Geometry: final body of the model. Coordinates: model frame, mm. A direction names the side the tool comes from. Coordinates: 2 decimals unless noted, no trailing zeros. Order: outer loops, then holes, each group sorted by start corner. A loop starts at its lowest first (then second) coordinate and runs counter-clockwise, first axis right, second up. Notation, with made-up numbers: M -34.75,5 L 20.25,5 A22 cw 20.25,18 Z; hole C 25,-34.75 d7. An arc over 180 degrees is marked long. Use CSV: the item, a comma, the result in double quotes. Start each with the question number.
Q1. Section query A-A, the plane x = -10. Output: boundary loops of the cut face in (y, z), and give its area (3 significant figures).
Q2. Section query D-D, the plane x = 0. State how many separate pieces and enclosed holes the cut face has, and give its area (3 significant figures).
Q3. Section query C-C, the plane z = -4. Output: boundary loops of the cut face in (x, y), and give its area (3 significant figures).
Q4. First-contact query: P1, Ø0.9, axis at x = 13, z = 0, coming from the +Y side (1 decimal); P2, Ø0.9, axis at x = 1, y = 1.5, coming from the -Z side; P3, Ø2, axis at x = 9, y = 2, coming from the -Z side; P4, Ø13, axis at x = 2.5, z = 13, coming from the -Y side. Flat tips, straight axial feed; report the tip coordinate or a pass-through.
Q5. Ray query, probe 1 along Z at (x, y) = (10, 0.3); probe 2 along Z at (x, y) = (3, 0.55); probe 3 along Y at (x, z) = (16, 3). Return the intervals inside material, ascending.
Q6. Access query for faces 1 (the face through (6, 2, -10)), 2 (the face through (-16.595, 1.371, 0.456)), 3 (the face through (0, 0.75, 14)), 4 (the face through (-1.08, -1.56, 4.88)), 5 (the face through (0, 0.75, -13)). Directions: +Z, -Z, +X, -X, +Y, -Y. A direction counts if a zero-diameter tool reaches every point of the face in a straight line with its end or side. Return the directions, or none.
Q7. Mould query, pull axis Z, two halves, no side actions, for faces 6 (the face through (-13.75, 1.37, -0.03)), 7 (the face through (2.2, -3, -2.2)), 8 (the face through (-0.098, 1.815, -15.744)), 9 (the face through (-22, 1, 0)). Classes: +Z half, -Z half, draft (parallel to the pull), parting line (faces both ways), or undercut.
Q8. Section query B-B, the plane z = 18. Output: boundary loops of the cut face in (x, y), and give its area (3 significant figures).
Autodesk Inventor part; units mm, degrees
ref_plane "YZ Plane" through (0, 0, 0) normal (1, 0, 0) x (0, 1, 0)
ref_plane "XZ Plane" through (0, 0, 0) normal (0, 1, 0) x (-1, 0, 0)
ref_plane "XY Plane" through (0, 0, 0) normal (0, 0, 1) x (1, 0, 0)
sketch "Sketch1" plane through (0, 0, 0) normal (0, 1, 0) x (-1, 0, 0)
  line L0 (6, -15) -> (6, -6)
  line L1 (16, -6) -> (16, 0)
  line L2 (6, -15) -> (0, -15)
  line L3 (16, -6) -> (6, -6)
  arc A0 (0, -21) -> (6, -15) centre (0, -15) ccw
  arc A1 (16, -6) -> (22, 0) centre (16, 0) ccw
  line L4 (6, 15) -> (6, 6)
  line L5 (16, 6) -> (16, 0)
  line L6 (6, 15) -> (0, 15)
  line L7 (16, 6) -> (6, 6)
  arc A2 (6, 15) -> (0, 21) centre (0, 15) ccw
  arc A3 (22, 0) -> (16, 6) centre (16, 0) ccw
  line L8 (-6, -15) -> (-6, -6)
  line L9 (-16, -6) -> (-16, 0)
  line L10 (-6, -15) -> (0, -15)
  line L11 (-16, -6) -> (-6, -6)
  arc A4 (-6, -15) -> (0, -21) centre (0, -15) ccw
  arc A5 (-22, 0) -> (-16, -6) centre (-16, 0) ccw
  line L12 (-16, 6) -> (-16, 0)
  arc A6 (-16, 6) -> (-22, 0) centre (-16, 0) ccw
  line L13 (-16, 6) -> (-6, 6)
  line L14 (-6, 15) -> (-6, 6)
  line L15 (-6, 15) -> (0, 15)
  arc A7 (0, 21) -> (-6, 15) centre (0, 15) ccw
  point P0 (0, 0)
  dimension "d0" = 16
  dimension "d1" = 15
extrude "Extrusion1" add sketch "Sketch1" along normal blind 2.85
sketch "Sketch2" plane through (0, 0, 0) normal (0, -1, 0) x (1, 0, 0)
  line L0 (-6, -15) -> (-6, -6)
  line L1 (-6, -6) -> (-6, -15)
  line L2 (6, -6) -> (6, -15)
  line L3 (6, -6) -> (6, -15)
  arc A0 (-6, -15) -> (6, -15) centre (0, -15) ccw
  line L4 (-6, -6) -> (6, -6)
  line L5 (-6, 15) -> (-6, 6)
  line L6 (6, 6) -> (6, 15)
  arc A1 (6, 15) -> (-6, 15) centre (0, 15) ccw
  line L7 (-6, 6) -> (6, 6)
  point P0 (0, 0)
extrude "Extrusion2" cut sketch "Sketch2" against normal blind 1.45
sketch "Sketch3" plane through (0, 2.85, 0) normal (0, 1, 0) x (1, 0, 0)
  circle A0 centre (16, 0) radius 0.75
  circle A1 centre (0, -15) radius 0.75
  circle A2 centre (10, 0) radius 0.75
  circle A3 centre (13, 0) radius 0.75
  circle A4 centre (19, 0) radius 0.75
  arc A5 (6, 15) -> (-6, 15) centre (0, 15) ccw
  arc A6 (-6, -15) -> (6, -15) centre (0, -15) ccw
  circle A7 centre (-16, 0) radius 0.75
  circle A8 centre (-10, 0) radius 0.75
  circle A9 centre (-13, 0) radius 0.75
  circle A10 centre (-19, 0) radius 0.75
  circle A11 centre (0, -12) radius 0.75
  circle A12 centre (0, -18) radius 0.75
  arc A13 (16, -6) -> (16, 6) centre (16, 0) ccw
  arc A14 (-16, 6) -> (-16, -6) centre (-16, 0) ccw
  circle A15 centre (0, 15) radius 0.75
  circle A16 centre (0, 12) radius 0.75
  circle A17 centre (0, 18) radius 0.75
  point P0 (0, 0)
  dimension "d10" = 1.5
  dimension "d12" = 1.5
  dimension "d14" = 1.5
  dimension "d17" = 1.5
  dimension "d19" = 1.5
  dimension "d22" = 1.5
extrude "Extrusion3" cut sketch "Sketch3" against normal blind 2.85
sketch "Sketch4" plane through (0, 2.85, 0) normal (0, 1, 0) x (1, 0, 0)
  circle A0 centre (0, 0) radius 3
  dimension "d25" = 6
extrude "Extrusion4" cut sketch "Sketch4" against normal blind 1.4
sketch "Sketch5" plane through (0, 1.45, 0) normal (0, 1, 0) x (1, 0, 0)
  circle A0 centre (0, 0) radius 1.35
  dimension "d28" = 2.7
extrude "Extrusion5" cut sketch "Sketch5" against normal blind 1.45
sketch "Sketch6" plane through (0, 1.45, 0) normal (0, -1, 0) x (1, 0, 0)
  circle A0 centre (0, 18) radius 0.75
  circle A1 centre (0, 12) radius 0.75
  circle A2 centre (0, 15) radius 0.75
  line L0 (6, 6) -> (-6, 6)
  line L1 (6, 15) -> (6, 6)
  arc A3 (6, 15) -> (-6, 15) centre (0, 15) ccw
  line L2 (-6, 6) -> (-6, 15)
  point P0 (0, 0)
extrude "Extrusion6" add sketch "Sketch6" along normal blind 0.7
sketch "Sketch7" plane through (0, 1.45, 0) normal (0, -1, 0) x (1, 0, 0)
  circle A0 centre (0, -18) radius 0.75
  circle A1 centre (0, -15) radius 0.75
  circle A2 centre (0, -12) radius 0.75
  line L0 (6, -6) -> (6, -15)
  line L1 (-6, -6) -> (6, -6)
  line L2 (-6, -15) -> (-6, -6)
  arc A3 (-6, -15) -> (6, -15) centre (0, -15) ccw
  point P0 (0, 0)
extrude "Extrusion7" add sketch "Sketch7" along normal blind 0.7
sketch "Sketch8" plane through (0, 0, 0) normal (0, -1, 0) x (1, 0, 0)
  circle A0 centre (0, 0) radius 1.35
  circle A1 centre (13, 0) radius 0.75
  circle A2 centre (-19, 0) radius 0.75
  circle A3 centre (-16, 0) radius 0.75
  circle A4 centre (16, 0) radius 0.75
  circle A5 centre (10, 0) radius 0.75
  circle A6 centre (-10, 0) radius 0.75
  circle A7 centre (-13, 0) radius 0.75
  circle A8 centre (19, 0) radius 0.75
  line L0 (-16, 6) -> (16, 6)
  arc A9 (-16, 6) -> (-16, -6) centre (-16, 0) ccw
  line L1 (16, -6) -> (-16, -6)
  arc A10 (16, -6) -> (16, 6) centre (16, 0) ccw
extrude "Extrusion8" add sketch "Sketch8" along normal blind 0.15
sketch "Sketch9" plane through (0, -0.15, 0) normal (0, -1, 0) x (1, 0, 0)
  circle A0 centre (0, 0) radius 5
  dimension "d37" = 10
extrude "Extrusion9" add sketch "Sketch9" along normal blind 2.85
sketch "Sketch10" plane through (0, -3, 0) normal (0, -1, 0) x (1, 0, 0)
  circle A0 centre (0, 0) radius 2.75
  dimension "d40" = 5.5
extrude "Extrusion10" cut sketch "Sketch10" against normal blind 2.85
properties part number "MMAE 232 Assignment 2_Servo Horn 3 - Dylan Tamras"
Responses:
1,outline,"M -0.15,-6 L 2.85,-6 L 2.85,-0.75 L -0.15,-0.75 Z; M -0.15,0.75 L 2.85,0.75 L 2.85,6 L -0.15,6 Z"
1,area,"31.5 mm²"
2,separate pieces,"8"
2,enclosed holes,"0"
2,area,"80.2 mm²"
3,outline,"M -20.47,-0.15 L -3,-0.15 L -3,-3 L 3,-3 L 3,-0.15 L 20.47,-0.15 L 20.47,2.85 L -20.47,2.85 Z"
3,area,"140 mm²"
4,P1,"passes through"
4,P2,"stops at z = -20.97"
4,P3,"stops at z = -6"
4,P4,"stops at y = 0.75"
5,probe 1,"z = -6 to -0.75, 0.75 to 6"
5,probe 2,"z = -6 to 6"
5,probe 3,"y = -0.15 to 2.85"
6,face 1,"-Z, +X, +Y, -Y"
6,face 2,"+Y, -Y"
6,face 3,"+Z, +X, -X, -Y"
6,face 4,"-Y"
6,face 5,"-Z, +X, -X, -Y"
7,face 6,"undercut"
7,face 7,"draft"
7,face 8,"undercut"
7,face 9,"parting line"
8,outline,"M -5.2,0.75 L -0.75,0.75 L -0.75,2.85 L -5.2,2.85 Z; M 0.75,0.75 L 5.2,0.75 L 5.2,2.85 L 0.75,2.85 Z"
8,area,"18.7 mm²"
